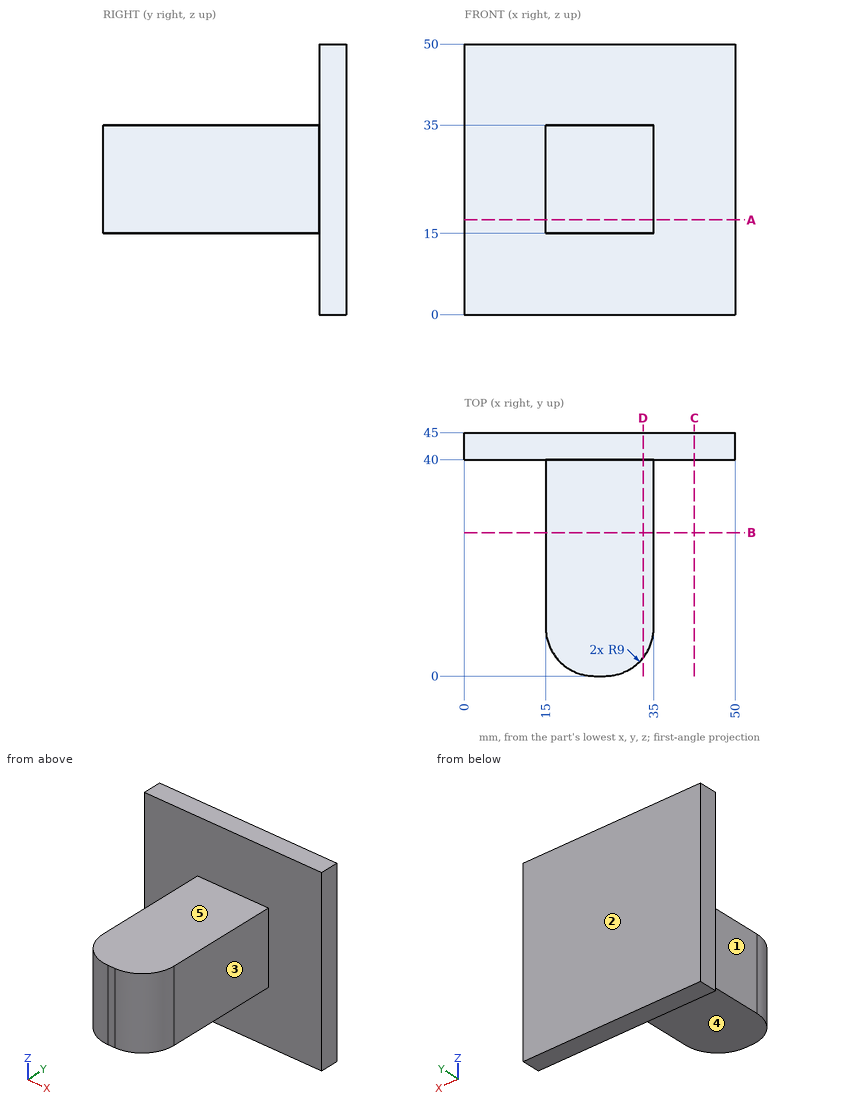
Job drawing, mm, ordinate dimensions from the low corner. One solid piece. A direction names the side the tool comes from. Round coordinates to 2 decimals unless told otherwise and drop trailing zeros. Loops run counter-clockwise (first coordinate to the right, second up) from the corner with the lowest first, then second, coordinate; pieces in that order, holes last. Notation, with made-up numbers: M 71,-24 L 122,-24 A17 cw 122,-17 Z; hole C 32,69 d3. An arc over 180 degrees is marked long. One line per question, with ' | ' between items. Start each with the question number.
Item 1: Wall check: line 1 (Y direction, x = 18, z = 4); line 2 (X direction, y = 39.5, z = 25). Give the ranges that are in metal, low to high.
Item 2: Cut at C-C, the plane x = 42.5. Write the cut outline in (y, z), plus the area to 3 significant figures.
Item 3: Cut at A-A, the plane z = 17.5. Write the cut outline in (x, y), plus the area to 3 significant figures.
Item 4: Cut at D-D, the plane x = 33. Write the cut outline in (y, z), plus the area to 3 significant figures.
Item 5: Which spindle directions (+Z, -Z, +X, -X, +Y, -Y) get a long thin tool onto all of the face, cutting with end or side? Do the marked faces 1, 2, 3, 4 and 5. Say none if no direction does.
Item 6: Pin check, flat tips, straight feed: pin 1 Ø10 at (x, y) = (29.5, 5) entering from -Z; pin 2 Ø16 at (y, z) = (17, 29.5) entering from -X; pin 3 Ø16 at (x, y) = (29, 16) entering from +Z. Stop position of each tip, or through.
Item 7: Cut at B-B, the plane y = 26.5. Write the cut outline in (x, z).
Responses:
1) line 1: y = 40 to 45 | line 2: x = 15 to 35
2) outline: M 40,0 L 45,0 L 45,50 L 40,50 Z | area: 250 mm²
3) outline: M 0,40 L 15,40 L 15,9 A9 ccw 24,0 L 26,0 A9 ccw 35,9 L 35,40 L 50,40 L 50,45 L 0,45 Z | area: 1,020 mm²
4) outline: M 3.34,15 L 40,15 L 40,0 L 45,0 L 45,50 L 40,50 L 40,35 L 3.34,35 Z | area: 983 mm²
5) face 1: +Z, -Z, -X, -Y | face 2: +Z, -Z, +X, -X, +Y | face 3: +Z, -Z, +X, -Y | face 4: -Z, +X, -X, -Y | face 5: +Z, +X, -X, -Y
6) pin 1: stops at z = 15 | pin 2: stops at x = 15 | pin 3: stops at z = 35
7) outline: M 15,15 L 35,15 L 35,35 L 15,35 Z
